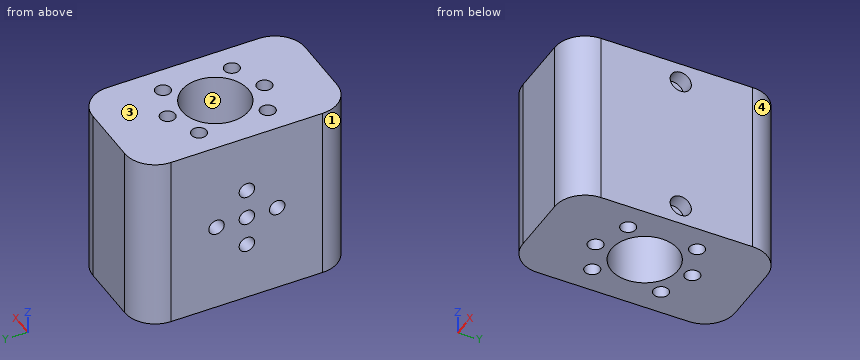
```python
from build123d import *

# Parameters (mm, degrees)
SKETCH1_W           = 40
SKETCH1_H           = 70
BOSS_EXTRUDE1_DEPTH = 59
SKETCH2_R           = 11
SKETCH2_R_2         = 2.5
CUT_EXTRUDE1_DEPTH  = 72.504101247
SKETCH5_R           = 2.55
CUT_EXTRUDE3_DEPTH  = 5
FILLET1_R           = 10
FILLET2_R           = 10
FILLET3_R           = 10
FILLET4_R           = 10
CUT_EXTRUDE4_START  = 20.060831
SKETCH10_R          = 3.5
CUT_EXTRUDE4_DEPTH  = 5


with BuildPart() as part:
    # Sketch1 → Boss-Extrude1 (new body)
    with BuildSketch(Plane.XY):
        with Locations((0.060830656, 0.062794648)):
            Rectangle(SKETCH1_W, SKETCH1_H)
    extrude(amount=BOSS_EXTRUDE1_DEPTH)

    # Sketch2 → Cut-Extrude1 (cut, through all)
    with BuildSketch(Plane.XY):
        Circle(SKETCH2_R)
        with Locations((-11.313708499, 11.313708499)):
            Circle(SKETCH2_R_2)
        with Locations((-0.122338904, 15.759725587)):
            Circle(SKETCH2_R_2)
        with Locations((11.402693442, 11.263696484)):
            Circle(SKETCH2_R_2)
        with Locations((11.339369089, -11.406422087)):
            Circle(SKETCH2_R_2)
        with Locations((-0.312311964, -16.029099896)):
            Circle(SKETCH2_R_2)
        with Locations((-11.204100775, -11.406422087)):
            Circle(SKETCH2_R_2)
    extrude(amount=CUT_EXTRUDE1_DEPTH, mode=Mode.SUBTRACT)

    # Sketch5 → Cut-Extrude3 (cut)
    with BuildSketch(Plane.ZY.offset(19.939169344)):
        with Locations((29.5, 0.062794648)):
            Circle(SKETCH5_R)
        with Locations((39.5, 0.062794648)):
            Circle(SKETCH5_R)
        with Locations((19.5, 0.062794648)):
            Circle(SKETCH5_R)
        with Locations((29.5, 10.062794648)):
            Circle(SKETCH5_R)
        with Locations((29.5, -9.937205352)):
            Circle(SKETCH5_R)
    extrude(amount=-CUT_EXTRUDE3_DEPTH, mode=Mode.SUBTRACT)

    # Fillet1
    fillet1_edges = [part.edges().sort_by_distance(p)[0] for p in [
        (20.060830656, 35.062794648, 29.5),
    ]]
    fillet(fillet1_edges, radius=FILLET1_R)

    # Fillet2
    fillet2_edges = [part.edges().sort_by_distance(p)[0] for p in [
        (20.060830656, -34.937205352, 29.5),
    ]]
    fillet(fillet2_edges, radius=FILLET2_R)

    # Fillet3
    fillet3_edges = [part.edges().sort_by_distance(p)[0] for p in [
        (-19.939169344, -34.937205352, 29.5),
    ]]
    fillet(fillet3_edges, radius=FILLET3_R)

    # Fillet4
    fillet4_edges = [part.edges().sort_by_distance(p)[0] for p in [
        (-19.939169344, 35.062794648, 29.5),
    ]]
    fillet(fillet4_edges, radius=FILLET4_R)

    # Sketch10 → Cut-Extrude4 (cut)
    with BuildSketch(Plane(origin=(0, 0, 0), x_dir=(0, 0, -1), z_dir=(1, 0, 0)).offset(CUT_EXTRUDE4_START)):
        with Locations((-52.5, 1.34000523)):
            Circle(SKETCH10_R)
        with Locations((-6.5, 1.34000523)):
            Circle(SKETCH10_R)
    extrude(amount=-CUT_EXTRUDE4_DEPTH, mode=Mode.SUBTRACT)


solid = part.part
```
Check sheet for the modelled part. Datum: model origin and axes. Units: mm. Face numbers are marked on the shaded views. Round coordinates to 2 decimals unless told otherwise and drop trailing zeros. Write each loop counter-clockwise with the first axis right and the second up, starting at its lowest first coordinate (ties: lowest second). Pieces come first, ordered by that corner, then holes. Notation, with made-up numbers: (2.25, 22) -> (7.25, 22) arc R37 ccw to (7.25, 59) -> close; hole circle Ø1 at (72.5, 63.5). An arc over 180 degrees is marked (long way). One line per question, with ' | ' between items. Start each with the question number.
1. Sectioned sample at C-C, the plane x = 0. Record the cut outline in (y, z), then the cut area to 3 significant figures.
2. Depth check by flat-ended pin: pin 1 (2.5 mm diameter, centred on y = 1, z = 40, fed in from -X); pin 2 (2 mm diameter, centred on y = 1.5, z = 7.5, fed in from +X). Enter the tip coordinate at first touch or a pass-through.
3. Sectioned sample at D-D, the plane z = 5. Record the cut outline in (x, y), then the cut area to 3 significant figures.
4. Sectioned sample at A-A, the plane z = 39.5. Record the cut outline in (x, y), then the cut area to 3 significant figures.
5. Release check for a two-part mould opening along Y. For the marked faces 1, 2, 3 and 4 record: +Y half, -Y half, draft (parallel to the pull), parting line (faces both ways), or undercut.
6. Sectioned sample at B-B, the plane x = -5. Record the cut outline in (y, z), then the cut area to 3 significant figures.
7. Scan lines: line 1 along X through (y, z) = (0, 39); line 2 along Y through (x, z) = (-12.5, 47); line 3 along Y through (x, z) = (-13, 7). Record each from-to range of solid material in increasing order. Write a range as from..to.
Taken from the geometry:
1) outline: (-34.94, 0) -> (-18.51, 0) -> (-18.51, 59) -> (-34.94, 59) -> close; (-13.55, 0) -> (-11, 0) -> (-11, 59) -> (-13.55, 59) -> close; (11, 0) -> (13.26, 0) -> (13.26, 59) -> (11, 59) -> close; (18.26, 0) -> (35.06, 0) -> (35.06, 59) -> (18.26, 59) -> close | area: 2,240 mm^2
2) pin 1: stops at x = -14.94 | pin 2: stops at x = 15.06
3) outline: (-19.94, -24.94) arc R10 ccw to (-9.94, -34.94) -> (10.06, -34.94) arc R10 ccw to (20.06, -24.94) -> (20.06, -1.82) -> (15.06, -1.82) -> (15.06, 4.5) -> (20.06, 4.5) -> (20.06, 25.06) arc R10 ccw to (10.06, 35.06) -> (-9.94, 35.06) arc R10 ccw to (-19.94, 25.06) -> close; hole circle Ø5 at (-11.31, 11.31); hole circle Ø5 at (-11.2, -11.41); hole circle Ø22 at (0, 0); hole circle Ø5 at (-0.31, -16.03); hole circle Ø5 at (-0.12, 15.76); hole circle Ø5 at (11.34, -11.41); hole circle Ø5 at (11.4, 11.26) | area: 2,180 mm^2
4) outline: (-19.94, -24.94) arc R10 ccw to (-9.94, -34.94) -> (10.06, -34.94) arc R10 ccw to (20.06, -24.94) -> (20.06, 25.06) arc R10 ccw to (10.06, 35.06) -> (-9.94, 35.06) arc R10 ccw to (-19.94, 25.06) -> (-19.94, 2.61) -> (-14.94, 2.61) -> (-14.94, -2.49) -> (-19.94, -2.49) -> close; hole circle Ø5 at (-11.31, 11.31); hole circle Ø5 at (-11.2, -11.41); hole circle Ø22 at (0, 0); hole circle Ø5 at (-0.31, -16.03); hole circle Ø5 at (-0.12, 15.76); hole circle Ø5 at (11.34, -11.41); hole circle Ø5 at (11.4, 11.26) | area: 2,190 mm^2
5) face 1: -Y half | face 2: undercut | face 3: draft | face 4: +Y half
6) outline: (-34.94, 0) -> (-9.8, 0) -> (-9.8, 59) -> (-34.94, 59) -> close; (9.8, 0) -> (35.06, 0) -> (35.06, 59) -> (9.8, 59) -> close | area: 2,970 mm^2
7) line 1: x = -14.94..-11, 11..20.06 | line 2: y = -34.6..-13.54, -9.27..9.11, 13.51..34.73 | line 3: y = -34.46..-13.15, -9.67..9.47, 13.16..34.58
